Input: part model. Units: mm. Frame: model coordinates. A direction names the side the tool comes from. Coordinates: 2 decimals unless noted, no trailing zeros. Write each loop counter-clockwise with the first axis right and the second up, starting at its lowest first coordinate (ties: lowest second). Pieces come first, ordered by that corner, then holes. Notation, with made-up numbers: M -27,25 L 1,25 A26 ccw 1,49 Z; hole C 26,12.25 d5. An arc over 180 degrees is marked long. Use one line per item in the form item = value.
from build123d import *

# Parameters (mm, degrees)
F1_DEPTH        = 10
F2_R            = 30
F3_DEPTH        = 30
F4_R            = 45
F4_R_2          = 30
F5_DEPTH        = 5
F6_R            = 4
F7_DEPTH        = 5
F8_R            = 4
F9_DEPTH        = 10.001
F11_D           = 5
F11_CSINK_D     = 32
F11_CSINK_ANGLE = 90


with BuildPart() as f1:
    # F0 (on Front) → F1 (new body)
    with BuildSketch(Plane.XZ):
        with BuildLine():
            Line((120, 40), (0, 40))
            ThreePointArc((0, 40), (-40, 0), (0, -40))
            Line((0, -40), (120, -40))
            Line((120, -40), (120, 40))
        make_face()
    extrude(amount=F1_DEPTH)

    # F2 (on face) → F3 (join)
    with BuildSketch(Plane.XZ.offset(10)):
        Circle(F2_R)
    extrude(amount=F3_DEPTH)

    # F4 (on face) → F5 (join)
    with BuildSketch(Plane.XZ.offset(40)):
        Circle(F4_R)
        Circle(F4_R_2, mode=Mode.SUBTRACT)
        Circle(F4_R_2)
    extrude(amount=F5_DEPTH)

    # F6 (on face) → F7 (cut, through all)
    with BuildSketch(Plane.XZ.offset(45)):
        with Locations((-19.3139053881, 33.4526654248)):
            Circle(F6_R)
        with Locations((19.3139053881, 33.4526654248)):
            Circle(F6_R)
        with Locations((38.6278107762, 0)):
            Circle(F6_R)
        with Locations((19.3139053881, -33.4526654248)):
            Circle(F6_R)
        with Locations((-19.3139053881, -33.4526654248)):
            Circle(F6_R)
        with Locations((-38.6278107762, 0)):
            Circle(F6_R)
    extrude(amount=-F7_DEPTH, mode=Mode.SUBTRACT)

    # F8 (on face) → F9 (cut, through all)
    with BuildSketch(Plane.XZ.offset(10)):
        with Locations((65, 22.5)):
            Circle(F8_R)
        with Locations((100, 22.5)):
            Circle(F8_R)
        with Locations((65, -22.5)):
            Circle(F8_R)
        with Locations((100, -22.5)):
            Circle(F8_R)
    extrude(amount=-F9_DEPTH, mode=Mode.SUBTRACT)

    # F11 (through all)
    with Locations(Plane.XZ.offset(45)):
        with Locations((0, 0)):
            CounterSinkHole(F11_D / 2, F11_CSINK_D / 2, counter_sink_angle=F11_CSINK_ANGLE)


solid = f1.part
(1) Line query: probe 1 along Z at (x, y) = (100, -3); probe 2 along Y at (x, z) = (17, -28); probe 3 along Z at (x, y) = (0, -12). Output: solid intervals per line, ascending.
Computed:
probe_1 = -40 to -26.5, -18.5 to 18.5, 26.5 to 40
probe_2 = -45 to -40, -10 to 0
probe_3 = -30 to -2.5, 2.5 to 30
(2) Set-up query: faces 5 (the flat face through (9, -40, -29)), 6 (the cylindrical face through (68.815, -5.07, 23.701)), 7 (the cylindrical face through (18.447, -42.535, 29.548)). Return all of +Z, -Z, +X, -X, +Y, -Y with unobstructed straight access to the full face (end or side cutting, diameter ignored); none if empty.
Computed:
face_5 = none
face_6 = +Y, -Y
face_7 = -Y
(3) Section query A-A on x = 100. Return the cut outline in (y, z).
Computed:
outline = M -10,-40 L 0,-40 L 0,-26.5 L -10,-26.5 Z; M -10,-18.5 L 0,-18.5 L 0,18.5 L -10,18.5 Z; M -10,26.5 L 0,26.5 L 0,40 L -10,40 Z
(4) Section query C-C on y = -28. Return the cut outline in (x, z), plus the area to 3 significant figures.
Computed:
outline = C 0,0 d60; hole C 0,0 d5
area = 2,810 mm^2
(5) First-contact query: pin 1 Ø5 at (x, y) = (29.5, -27) entering from -Z; pin 2 Ø7 at (x, z) = (65, 22.5) entering from -Y; pin 3 Ø10.5 at (x, z) = (100, 22.5) entering from -Y; pin 4 Ø1.5 at (x, y) = (15.5, -39) entering from +Z. Flat tips, straight axial feed; report the tip coordinate or a pass-through.
Computed:
pin_1 = -13.08
pin_2 = through
pin_3 = -10
pin_4 = 26.12
(6) Section query B-B on z = 0. Return the cut outline in (x, y), plus the area to 3 significant figures.
Computed:
outline = M -45,-45 L -42.63,-45 L -42.63,-40 L -45,-40 Z; M -40,-10 L -30,-10 L -30,-40 L -34.63,-40 L -34.63,-45 L -16,-45 L -2.5,-31.5 L -2.5,0 L -40,0 Z; M 2.5,-31.5 L 16,-45 L 34.63,-45 L 34.63,-40 L 30,-40 L 30,-10 L 120,-10 L 120,0 L 2.5,0 Z; M 42.63,-45 L 45,-45 L 45,-40 L 42.63,-40 Z
area = 3,360 mm^2
(7) Section query D-D on x = 33. Return the cut outline in (y, z), plus the area to 3 significant figures.
Computed:
outline = M -45,-30.59 L -40,-30.59 L -40,30.59 L -45,30.59 Z; M -10,-40 L 0,-40 L 0,40 L -10,40 Z
area = 1,110 mm^2
(8) Pull-direction query (X, two-part tool) for faces 1 (the flat face through (59, -5, -40)), 2 (the cylindrical face through (-39.99, -4.93, 0.88)), 3 (the cylindrical face through (-15.619, -42.535, -34.985)), 4 (the cylindrical face through (20.765, -42.465, -39.923)); classes: pulls with the +X half, pulls with the -X half, needs draft (parallel to the pull), parting line crosses it, or undercut.
Computed:
face_1 = needs draft
face_2 = pulls with the -X half
face_3 = undercut
face_4 = parting line crosses it
